Part model, mm, in its own coordinate system. A direction names the side the tool comes from. Round coordinates to 2 decimals unless told otherwise and drop trailing zeros. Loops run counter-clockwise (first coordinate to the right, second up) from the corner with the lowest first, then second, coordinate; pieces in that order, holes last. Notation, with made-up numbers: (76, 11.5) -> (134, 11.5) arc R10 cw to (134, 20.5) -> close; hole circle Ø3 at (33, 32.5). An arc over 180 degrees is marked (long way). Use a Markdown table: item, result. Add a question column.
Item 1: Flat gauge pins, fed straight in: pin 1 (8.5 mm diameter, centred on y = 4, z = -1.5, fed in from -X); pin 2 (1.5 mm diameter, centred on x = 3.5, y = -8.5, fed in from +Z); pin 3 (6 mm diameter, centred on y = 6.5, z = -1.5, fed in from +X) (3 decimals). Where does each tip first touch, or does it go through?
Item 2: Cut at D-D, the plane z = -17. List the corners of the cut face in (x, y).
Item 3: Probe line 1 (X direction, y = 1.5, z = -0.5); line 2 (Z direction, x = 1, y = -4); line 3 (Z direction, x = 2.5, y = -12). List the from-to ranges inside material, lowest first. Write a range as [from, to].
Item 4: Cut at A-A, the plane z = 0. List the corners of the cut face in (x, y) (1 decimal), plus the area to 3 significant figures.
Item 5: Which spindle directions (+Z, -Z, +X, -X, +Y, -Y) get a long thin tool onto all of the face, cutting with end or side? Do faces 1 (the face through (-20, 16.51, -11)), 2 (the face through (-5, 17.78, 5)), 3 (the face through (3.38, 0.249, -5.747)). Say none if no direction does.
Item 6: Two-plate mould, pull along X, no slides. Class faces 4 (the face through (-20, -16.51, -11)), 5 (the face through (-3.29, 0.25, -5.8)), 6 (the face through (7.248, -17.136, 23.016)), 7 (the face through (-3.38, 0.249, 5.747)): pulls with the +X half, pulls with the -X half, needs draft (parallel to the pull), parting line crosses it, or undercut.
Item 7: Cut at C-C, the plane x = 4.5. List the corners of the cut face in (y, z).
```python
from build123d import *

# Parameters (mm, degrees)
SKETCH1_R           = 24.13
BOSS_EXTRUDE1_DEPTH = 17.78
SKETCH2_W           = 3.81
SKETCH2_H           = 15.24


with BuildPart() as part:
    # Sketch1 → Boss-Extrude1 (new, symmetric)
    with BuildSketch(Plane(origin=(0, 0, 0), x_dir=(1, 0, 0), z_dir=(0, 1, 0))):
        with Locations(Location((0, 0, 0), (0, 0, 270))):
            Circle(SKETCH1_R)
        Polygon((0, 7.69896584), (-6.6675, 3.84948292), (-6.6675, -3.84948292), (0, -7.69896584), (6.6675, -3.84948292), (6.6675, 3.84948292), align=None, mode=Mode.SUBTRACT)
    extrude(amount=BOSS_EXTRUDE1_DEPTH, both=True)

    # Sketch2 → Cut-Revolve1 (revolve, cut)
    with BuildSketch(Plane.XY, mode=Mode.PRIVATE) as cut_revolve1_sk:
        with Locations((-24.13, 8.89)):
            Rectangle(SKETCH2_W, SKETCH2_H)
        with Locations((-24.13, -8.89)):
            Rectangle(SKETCH2_W, SKETCH2_H)
    revolve(cut_revolve1_sk.sketch.rotate(Axis((0, 17.78, 0), (0, -1, 0)), 90), axis=Axis((0, 17.78, 0), (0, -1, 0)), mode=Mode.SUBTRACT)


solid = part.part
```
A:
| question | item | result |
|---|---|---|
| 1 | pin 1 | stops at x = -24.13 |
| 1 | pin 2 | stops at z = 22.05 |
| 1 | pin 3 | stops at x = 22.225 |
| 2 | outline | (-17.12, -17.78) -> (17.12, -17.78) -> (17.12, -16.51) -> (14.32, -16.51) -> (14.32, -1.27) -> (17.12, -1.27) -> (17.12, 1.27) -> (14.32, 1.27) -> (14.32, 16.51) -> (17.12, 16.51) -> (17.12, 17.78) -> (-17.12, 17.78) -> (-17.12, 16.51) -> (-14.32, 16.51) -> (-14.32, 1.27) -> (-17.12, 1.27) -> (-17.12, -1.27) -> (-14.32, -1.27) -> (-14.32, -16.51) -> (-17.12, -16.51) -> close |
| 3 | line 1 | x = [-22.22, -6.67], [6.67, 22.22] |
| 3 | line 2 | z = [-22.2, -7.12], [7.12, 22.2] |
| 3 | line 3 | z = [-22.08, -6.26], [6.26, 22.08] |
| 4 | outline | (-24.1, -17.8) -> (-6.7, -17.8) -> (-6.7, 17.8) -> (-24.1, 17.8) -> (-24.1, 16.5) -> (-22.2, 16.5) -> (-22.2, 1.3) -> (-24.1, 1.3) -> (-24.1, -1.3) -> (-22.2, -1.3) -> (-22.2, -16.5) -> (-24.1, -16.5) -> close; (6.7, -17.8) -> (24.1, -17.8) -> (24.1, -16.5) -> (22.2, -16.5) -> (22.2, -1.3) -> (24.1, -1.3) -> (24.1, 1.3) -> (22.2, 1.3) -> (22.2, 16.5) -> (24.1, 16.5) -> (24.1, 17.8) -> (6.7, 17.8) -> close |
| 4 | area | 1,130 mm^2 |
| 5 | face 1 | none |
| 5 | face 2 | +Z, -Z, +X, -X, +Y |
| 5 | face 3 | +Y, -Y |
| 6 | face 4 | needs draft |
| 6 | face 5 | undercut |
| 6 | face 6 | parting line crosses it |
| 6 | face 7 | undercut |
| 7 | outline | (-17.78, -23.71) -> (-16.51, -23.71) -> (-16.51, -21.76) -> (-1.27, -21.76) -> (-1.27, -23.71) -> (1.27, -23.71) -> (1.27, -21.76) -> (16.51, -21.76) -> (16.51, -23.71) -> (17.78, -23.71) -> (17.78, -5.1) -> (-17.78, -5.1) -> close; (-17.78, 5.1) -> (17.78, 5.1) -> (17.78, 23.71) -> (16.51, 23.71) -> (16.51, 21.76) -> (1.27, 21.76) -> (1.27, 23.71) -> (-1.27, 23.71) -> (-1.27, 21.76) -> (-16.51, 21.76) -> (-16.51, 23.71) -> (-17.78, 23.71) -> close |
